from build123d import *

# Parameters (mm, degrees)
SKETCH1_W           = 131
SKETCH1_H           = 96
BOSS_EXTRUDE1_DEPTH = 1.5
SKETCH2_R           = 1.5
BOSS_EXTRUDE2_DEPTH = 3
CHAMFER1_SIZE       = 5
CUT_EXTRUDE1_DEPTH  = 15


with BuildPart() as part:
    # Sketch1 → Boss-Extrude1 (new, symmetric)
    with BuildSketch(Plane(origin=(0, 0, 0), x_dir=(1, 0, 0), z_dir=(0, 1, 0))):
        Rectangle(SKETCH1_W, SKETCH1_H)
    extrude(amount=BOSS_EXTRUDE1_DEPTH, both=True)

    # Sketch2 → Boss-Extrude2 (add)
    with BuildSketch(Plane.ZY.offset(65.5)):
        Polygon((-33, 16.5), (-48, 1.5), (0, 1.5), (0, 16.5), align=None)
        with Locations((-33.3, 11.5)):
            Circle(SKETCH2_R, mode=Mode.SUBTRACT)
        with Locations((-5.7, 11.5)):
            Circle(SKETCH2_R, mode=Mode.SUBTRACT)
    boss_extrude2 = extrude(amount=-BOSS_EXTRUDE2_DEPTH)

    # Mirror1: Boss-Extrude2 across plane
    add(boss_extrude2.mirror(Plane(origin=(0, 0, 0), x_dir=(0, 0, 1), z_dir=(1, 0, 0))))

    # Chamfer1
    chamfer1_edges = [part.edges().sort_by_distance(p)[0] for p in [
        (-62.5, 1.5, -24),
        (62.5, 1.5, -24),
    ]]
    chamfer(chamfer1_edges, length=CHAMFER1_SIZE)

    # Sketch3 → Cut-Extrude1 (cut)
    with BuildSketch(Plane.ZY.offset(65.5)):
        Polygon((-20, -1.5), (-20, 4.5), (-8, 16.5), (-20, 16.5), (-23, 16.5), (-35, 4.5), (-35, -1.5), align=None)
    extrude(amount=-CUT_EXTRUDE1_DEPTH, mode=Mode.SUBTRACT)


solid = part.part
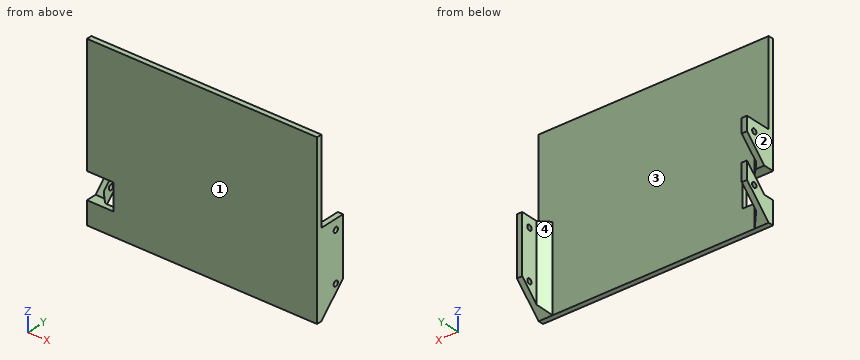
Read the model definition and answer for the solid it produces. Units are mm, in the model's axes. Face numbers are marked on the shaded views. Coordinates: 2 decimals unless noted, no trailing zeros. Loops run counter-clockwise (first coordinate to the right, second up) from the corner with the lowest first, then second, coordinate; pieces in that order, holes last. Notation, with made-up numbers: (-2.5, 25.25) -> (6.5, 25.25) arc R32 ccw to (6.5, 53.25) -> close; hole circle Ø11 at (19.5, -16). An arc over 180 degrees is marked (long way). Write item = value, one per line. Start each with the question number.
1) Given P1, Ø6.5, axis at x = -62, y = 12.5, coming from the +Z side; P2, Ø3, axis at x = -43.5, z = -2.5, coming from the +Y side; P3, Ø1.5, axis at y = -0.5, z = -26.5, coming from the -X side, each flat-ended and moving along its own axis, determine where each tip first touches the part or whether it passes through.
2) The part is cut by section C-C, the plane y = 3. Determine the outline of the cut face in (x, z).
3) The part is cut by section B-B, the plane y = 14.5. Determine the outline of the cut face in (x, z).
4) The part is cut by section A-A, the plane z = -5.7. Determine the outline of the cut face in (x, y), plus the area to 3 significant figures.
5) Find the intervals of material crossed by L1, parallel to X at y = 15, z = -30; L2, parallel to Y at x = 63, z = -33; L3, parallel to Y at x = -32, z = 9.5, in increasing order. Write a range as from..to.
6) The part is cut by section D-D, the plane x = 55. Determine the outline of the cut face in (y, z), plus the area to 3 significant figures.
7) The mould has two halves that part along X. Classify the marked faces 1, 2, 3 and 4: pulls with the +X half, pulls with the -X half, needs draft (parallel to the pull), parting line crosses it, or undercut.
Result:
q1.P1 = 0
q1.P2 = 1.5
q1.P3 = -50.5
q2.outline = (-65.5, -46.5) -> (-59, -46.5) -> (-59, -35) -> (-65.5, -35) -> close; (-65.5, -20) -> (-59, -20) -> (-59, 0) -> (-65.5, 0) -> close; (59, -46.5) -> (65.5, -46.5) -> (65.5, 0) -> (59, 0) -> close
q3.outline = (-65.5, -35) -> (-62.5, -35) -> (-62.5, -25) -> (-65.5, -25) -> close; (-65.5, -10) -> (-62.5, -10) -> (-62.5, 0) -> (-65.5, 0) -> close; (62.5, -35) -> (65.5, -35) -> (65.5, 0) -> (62.5, 0) -> close
q4.outline = (-65.5, -1.5) -> (65.5, -1.5) -> (65.5, 10) -> (62.5, 10) -> (62.5, 6.5) -> (57.5, 1.5) -> (-57.5, 1.5) -> (-62.5, 6.5) -> (-62.5, 10) -> (-65.5, 10) -> close; (-65.5, 13) -> (-62.5, 13) -> (-62.5, 16.5) -> (-65.5, 16.5) -> close; (62.5, 13) -> (65.5, 13) -> (65.5, 16.5) -> (62.5, 16.5) -> close
q4.area = 490 mm²
q5.L1 = -65.5..-62.5, 62.5..65.5
q5.L2 = -1.5..10.03, 12.97..16.5
q5.L3 = -1.5..1.5
q6.outline = (-1.5, -48) -> (1.5, -48) -> (1.5, 48) -> (-1.5, 48) -> close
q6.area = 288 mm²
q7.face_1 = needs draft
q7.face_2 = pulls with the -X half
q7.face_3 = undercut
q7.face_4 = undercut
